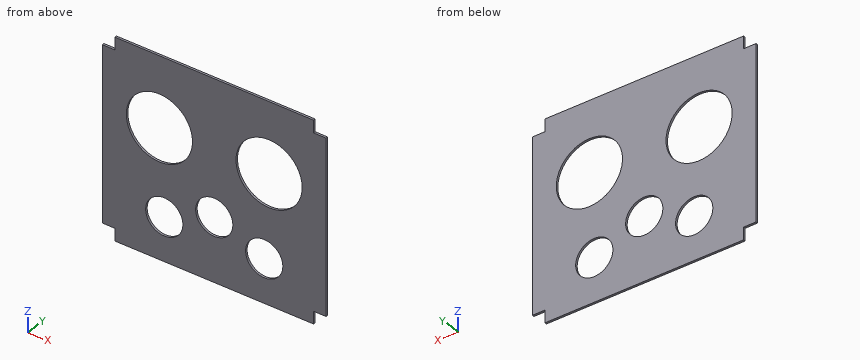
from build123d import *

# Parameters (mm, degrees)
SKETCH1_R           = 101.6
SKETCH1_R_2         = 57.15
BOSS_EXTRUDE1_DEPTH = 6.35


with BuildPart() as part:
    # Sketch1 → Boss-Extrude1 (new body)
    with BuildSketch(Plane(origin=(0, 0, 0), x_dir=(1, 0, 0), z_dir=(0, 1, 0))):
        Polygon((0, 0), (0, -38.1), (-609.6, -38.1), (-609.6, 0), (-647.7, 0), (-647.7, 533.4), (-609.6, 533.4), (-609.6, 571.5), (0, 571.5), (0, 533.4), (38.1, 533.4), (38.1, 0), align=None)
        with Locations((-473.075, 177.8)):
            Circle(SKETCH1_R, mode=Mode.SUBTRACT)
        with Locations((-136.525, 177.8)):
            Circle(SKETCH1_R, mode=Mode.SUBTRACT)
        with Locations((-304.8, 376.459625679)):
            Circle(SKETCH1_R_2, mode=Mode.SUBTRACT)
        with Locations((-151.485932589, 437.719781848)):
            Circle(SKETCH1_R_2, mode=Mode.SUBTRACT)
        with Locations((-458.114067411, 437.719781848)):
            Circle(SKETCH1_R_2, mode=Mode.SUBTRACT)
    extrude(amount=BOSS_EXTRUDE1_DEPTH)


solid = part.part
Source: CAD feature listing. Evaluate the final solid. Frame: model axes, mm. Round coordinates to 2 decimals unless told otherwise and drop trailing zeros. Loops run counter-clockwise (first coordinate to the right, second up) from the corner with the lowest first, then second, coordinate; pieces in that order, holes last. Notation, with made-up numbers: (14.5, 58) -> (24.5, 58) arc R20 cw to (24.5, 95) -> close; hole circle Ø7 at (0, -10). An arc over 180 degrees is marked (long way). Answer as a JSON object with one key per item and string values. Group by question number.
Q1. Ray query, line 1 (X direction, y = 2.25, z = -177.8) (3 decimals); line 2 (X direction, y = 4.25, z = -152.5); line 3 (Z direction, x = -135, y = 2.25). Return the intervals inside material, ascending. Write a range as from..to.
Q2. Section query D-D (y = 5.25). Output: boundary loops of the cut face in (x, z) (3 decimals), plus the area to 3 significant figures.
Q3. Contact query for flat-ended pins moving along their axis: P1, Ø1.9, axis at y = 4, z = -549.5, coming from the -X side; P2, Ø3, axis at x = 16.5, y = 3, coming from the -Z side; P3, Ø5, axis at x = -256, z = -354.5, coming from the +Y side. Output: stop coordinate, or through.
Q4. Section query A-A (z = -177.8). Output: boundary loops of the cut face in (x, y) (3 decimals).
Q5. Section query C-C (x = -113.5). Output: boundary loops of the cut face in (y, z).
Q6. Section query B-B (x = -304.8). Output: boundary loops of the cut face in (y, z), plus the area to 3 significant figures.
Completed:
{
 "1": {"line 1": "-647.7..-574.675, -371.475..-238.125, -34.925..38.1", "line 2": "-647.7..-571.47, -374.68..-234.92, -38.13..38.1", "line 3": "-571.5..-492.44, -383..-279.39, -76.21..38.1"},
 "2": {"outline": "(-647.7, -533.4) -> (-609.6, -533.4) -> (-609.6, -571.5) -> (0, -571.5) -> (0, -533.4) -> (38.1, -533.4) -> (38.1, 0) -> (0, 0) -> (0, 38.1) -> (-609.6, 38.1) -> (-609.6, 0) -> (-647.7, 0) -> close; hole circle Ø203.2 at (-473.075, -177.8); hole circle Ø114.3 at (-458.114, -437.72); hole circle Ø114.3 at (-304.8, -376.46); hole circle Ø203.2 at (-136.525, -177.8); hole circle Ø114.3 at (-151.486, -437.72)", "area": "317,000 mm²"},
 "3": {"P1": "x = -609.6", "P2": "z = -533.4", "P3": "through"},
 "4": {"outline": "(-647.7, 0) -> (-574.675, 0) -> (-574.675, 6.35) -> (-647.7, 6.35) -> close; (-371.475, 0) -> (-238.125, 0) -> (-238.125, 6.35) -> (-371.475, 6.35) -> close; (-34.925, 0) -> (38.1, 0) -> (38.1, 6.35) -> (-34.925, 6.35) -> close"},
 "5": {"outline": "(0, -571.5) -> (6.35, -571.5) -> (6.35, -480.42) -> (0, -480.42) -> close; (0, -395.02) -> (6.35, -395.02) -> (6.35, -276.76) -> (0, -276.76) -> close; (0, -78.84) -> (6.35, -78.84) -> (6.35, 38.1) -> (0, 38.1) -> close"},
 "6": {"outline": "(0, -571.5) -> (6.35, -571.5) -> (6.35, -433.61) -> (0, -433.61) -> close; (0, -319.31) -> (6.35, -319.31) -> (6.35, 38.1) -> (0, 38.1) -> close", "area": "3,150 mm²"}
}
